```python
from build123d import *

# Parameters (mm, degrees)
F0_W     = 40.64
F0_H     = 40.64
F0_R     = 9.665554
F1_DEPTH = 40.64
F2_R     = 9.652
F3_DEPTH = 40.641


with BuildPart() as f1:
    # F0 (on Front) → F1 (new body)
    with BuildSketch(Plane.XZ):
        with Locations((-20.32, 20.32)):
            Rectangle(F0_W, F0_H)
        with Locations((-20.32, 20.32)):
            Circle(F0_R, mode=Mode.SUBTRACT)
    extrude(amount=F1_DEPTH)

    # F2 (on face) → F3 (cut, through all)
    with BuildSketch(Plane.YZ):
        with Locations((-20.32, 20.32)):
            Circle(F2_R)
    extrude(amount=-F3_DEPTH, mode=Mode.SUBTRACT)


solid = f1.part
```
CAD build for the part. Positions are in the model's coordinates, mm. Round coordinates to 2 decimals unless told otherwise and drop trailing zeros. Write each loop counter-clockwise with the first axis right and the second up, starting at its lowest first coordinate (ties: lowest second). Pieces come first, ordered by that corner, then holes. Notation, with made-up numbers: M 36,87 L 60,87 A13 ccw 60,109 Z; hole C 28.25,12 d9. An arc over 180 degrees is marked long. One line per question, with ' | ' between items.
1. Cut at A-A on y = -20.32. Write the cut outline in (x, z), and give its area (3 significant figures).
Working result:
outline: M -40.64,0 L 0,0 L 0,10.67 L -19.81,10.67 A9.67 cw -20.83,10.67 L -40.64,10.67 Z; M -40.64,29.97 L -20.83,29.97 A9.67 cw -19.81,29.97 L 0,29.97 L 0,40.64 L -40.64,40.64 Z | area: 867 mm2
2. Cut at B-B on z = 20.32. Write the cut outline in (x, y).
Working result:
outline: M -40.64,-40.64 L -29.99,-40.64 L -29.99,-29.97 L -40.64,-29.97 Z; M -40.64,-10.67 L -29.99,-10.67 L -29.99,0 L -40.64,0 Z; M -10.65,-40.64 L 0,-40.64 L 0,-29.97 L -10.65,-29.97 Z; M -10.65,-10.67 L 0,-10.67 L 0,0 L -10.65,0 Z
3. Probe L1, parallel to Z at x = -20, y = -29; L2, parallel to Y at x = -10, z = 20.32; L3, parallel to Z at x = -29, y = -19. List the from-to ranges inside material, lowest first. Write a range as from..to.
Working result:
L1: 0..10.66, 29.98..40.64 | L2: -40.64..-29.97, -10.67..0 | L3: 0..10.76, 29.88..40.64
4. Mould opens along Z. For faces 1 (the cylindrical face through (-22.415, -15.52, 10.884)), 2 (the flat face through (-25, 0, 30)), 3 (the flat face through (-21, -20, 0)) say: pulls with the +Z half, pulls with the -Z half, needs draft (parallel to the pull), parting line crosses it, or undercut.
Working result:
face 1: undercut | face 2: needs draft | face 3: pulls with the -Z half
5. Cut at D-D on x = -32.5. Write the cut outline in (y, z), and give its area (3 significant figures).
Working result:
outline: M -40.64,0 L 0,0 L 0,40.64 L -40.64,40.64 Z; hole C -20.32,20.32 d19.3 | area: 1,360 mm2
6. Cut at C-C on y = -38. Write the cut outline in (x, z).
Working result:
outline: M -40.64,0 L 0,0 L 0,40.64 L -40.64,40.64 Z; hole C -20.32,20.32 d19.33
7. Pin check, flat tip, straight feed: pin 1 Ø12 at (x, y) = (-15, -26.5) entering from -Z. Stop position of the tip, or through.
Working result:
pin 1: z = 0
